Model file for the job. Use its own axes, mm. Face numbers are marked on the shaded views. A direction names the side the tool comes from. Give positions to 0.01 mm unless a question says otherwise; leave off trailing zeros. Write each loop counter-clockwise with the first axis right and the second up, starting at its lowest first coordinate (ties: lowest second). Pieces come first, ordered by that corner, then holes.
```python
from build123d import *

# Parameters (mm, degrees)
SKETCH_1_W          = 330
SKETCH_1_H          = 80
EXTRUDE_1_DEPTH     = 5
SKETCH_2_R          = 5.25
CUT_EXTRUDE_1_DEPTH = 5
SKETCH_3_R          = 4
CUT_EXTRUDE_2_DEPTH = 10
FILLET_1_R          = 10
SKETCH_13_R         = 6.969385005
EXTRUDE_5_DEPTH     = 5
SKETCH_14_W         = 5
SKETCH_14_H         = 75
EXTRUDE_6_DEPTH     = 80
SKETCH_15_W         = 20
SKETCH_15_H         = 5
EXTRUDE_7_DEPTH     = 80
EXTRUDE_8_DEPTH     = 5
SKETCH_17_R         = 3
CUT_EXTRUDE_5_DEPTH = 5
FILLET_2_R          = 1


with BuildPart() as part:
    # 草图1 → 凸台-拉伸1 (new body)
    with BuildSketch(Plane.XY):
        Rectangle(SKETCH_1_W, SKETCH_1_H)
    extrude(amount=EXTRUDE_1_DEPTH)

    # 草图2 → 切除-拉伸1 (cut)
    with BuildSketch(Plane.XY.offset(5)):
        with Locations((-145, 0)):
            Circle(SKETCH_2_R)
    extrude(amount=-CUT_EXTRUDE_1_DEPTH, mode=Mode.SUBTRACT)

    # 草图3 → 切除-拉伸2 (cut)
    with BuildSketch(Plane.XY.offset(5)):
        with Locations((-45, 0)):
            Circle(SKETCH_3_R)
    extrude(amount=-CUT_EXTRUDE_2_DEPTH, mode=Mode.SUBTRACT)

    # 圆角1
    fillet_1_edges = [part.edges().sort_by_distance(p)[0] for p in [
        (-165, 40, 2.5),
        (-165, -40, 2.5),
    ]]
    fillet(fillet_1_edges, radius=FILLET_1_R)

    # 草图13 → 凸台-拉伸5 (add)
    with BuildSketch(Plane.XY.offset(5)):
        with Locations((-45, 0)):
            Circle(SKETCH_13_R)
    extrude(amount=-EXTRUDE_5_DEPTH)

    # 草图14 → 凸台-拉伸6 (add)
    with BuildSketch(Plane.XZ.offset(40)):
        with Locations((162.5, -37.5)):
            Rectangle(SKETCH_14_W, SKETCH_14_H)
    extrude(amount=-EXTRUDE_6_DEPTH)

    # 草图15 → 凸台-拉伸7 (add)
    with BuildSketch(Plane.XZ.offset(40)):
        with Locations((150, -72.5)):
            Rectangle(SKETCH_15_W, SKETCH_15_H)
    extrude(amount=-EXTRUDE_7_DEPTH)

    # 草图16 → 凸台-拉伸8 (add)
    with BuildSketch(Plane.XZ.offset(40)):
        Polygon((5, 5), (5, 0), (140, -75), (165, -75), (165, 5), align=None)
    extrude_8 = extrude(amount=-EXTRUDE_8_DEPTH)

    # 镜向1: 凸台-拉伸8 across plane
    add(extrude_8.mirror(Plane.ZX))

    # 草图17 → 切除-拉伸5 (cut)
    with BuildSketch(Plane(origin=(0, 0, -75), x_dir=(-1, 0, 0), z_dir=(0, 0, -1))):
        with Locations((-152, -15)):
            Circle(SKETCH_17_R)
        with Locations((-152, 15)):
            Circle(SKETCH_17_R)
    extrude(amount=-CUT_EXTRUDE_5_DEPTH, mode=Mode.SUBTRACT)

    # 圆角2
    fillet_2_edges = [part.edges().sort_by_distance(p)[0] for p in [
        (72.5, 40, -37.5),
        (72.5, 35, -37.5),
        (165, 0, 5),
        (5, 40, 5),
        (-75, -40, 0),
        (5, -40, 5),
        (-165, 0, 0),
        (-162.071067812, 37.071067812, 0),
        (-162.071067812, -37.071067812, 0),
        (-165, 0, 5),
        (-162.071067812, 37.071067812, 5),
        (-162.071067812, -37.071067812, 5),
        (165, 0, -75),
        (152.5, -40, -75),
        (152.5, 40, -75),
        (72.5, -40, -37.5),
        (72.5, -35, -37.5),
        (165, 40, -35),
        (165, -40, -35),
        (-75, 40, 0),
    ]]
    fillet(fillet_2_edges, radius=FILLET_2_R)


solid = part.part
```
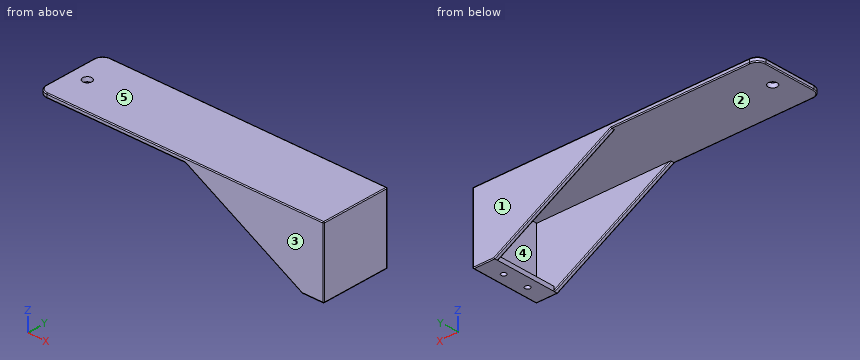
1. Pull direction Y, two halves, no side cores. Call the marked faces 1, 2 and 3: +Y half, -Y half, draft (parallel to the pull), parting line (faces both ways), or undercut.
Calculated:
face 1: +Y half
face 2: undercut
face 3: -Y half
2. Slice it at C-C, the plane x = -145. Write the cut outline in (y, z), and give its area (3 significant figures).
Calculated:
outline: (-40, 1) arc R1 ccw to (-39, 0) - (-5.25, 0) - (-5.25, 5) - (-39, 5) arc R1 ccw to (-40, 4) - close; (5.25, 0) - (39, 0) arc R1 ccw to (40, 1) - (40, 4) arc R1 ccw to (39, 5) - (5.25, 5) - close
area: 347 mm2
3. Pin check, flat tips, straight feed: P1, Ø4, axis at x = 83.5, y = 3.5, coming from the -Z side; P2, Ø8, axis at y = 9.5, z = -10, coming from the -X side; P3, Ø5.5, axis at y = 8, z = -72, coming from the -X side. Stop position of each tip, or through.
Calculated:
P1: stops at z = 0
P2: stops at x = 160
P3: stops at x = 140
4. Which spindle directions (+Z, -Z, +X, -X, +Y, -Y) get a long thin tool onto all of the face, cutting with end or side? Do the marked faces 4 and 5. Say none if no direction does.
Calculated:
face 4: -X
face 5: +Z, +X, -X, +Y, -Y
5. Probe probe 1 along Y at (x, z) = (152, -73.4); probe 2 along Y at (x, z) = (-145, 2.95); probe 3 along X at (y, z) = (23, -8). List the from-to ranges inside material, lowest first.
Calculated:
probe 1: y = -40 to -18, -12 to 12, 18 to 40
probe 2: y = -40 to -5.25, 5.25 to 40
probe 3: x = 160 to 165
6. Slice it at B-B, the plane y = 15. Write the cut outline in (x, z).
Calculated:
outline: (-165, 1) arc R1 ccw to (-164, 0) - (160, 0) - (160, -70) - (155, -70) - (155, -75) - (164, -75) arc R1 ccw to (165, -74) - (165, 4) arc R1 ccw to (164, 5) - (-164, 5) arc R1 ccw to (-165, 4) - close; (140, -75) - (149, -75) - (149, -70) - (140, -70) - close
7. Slice it at A-A, the plane x = 152. Write the cut outline in (y, z).
Calculated:
outline: (-40, -74) arc R1 ccw to (-39, -75) - (-18, -75) - (-18, -70) - (-35, -70) - (-35, 0) - (35, 0) - (35, -70) - (18, -70) - (18, -75) - (39, -75) arc R1 ccw to (40, -74) - (40, 4) arc R1 ccw to (39, 5) - (-39, 5) arc R1 ccw to (-40, 4) - close; (-12, -75) - (12, -75) - (12, -70) - (-12, -70) - close
